Source: CAD feature listing. Evaluate the final solid. Frame: model axes, mm. Give positions to 0.01 mm unless a question says otherwise; leave off trailing zeros. Order: outer loops, then holes, each group sorted by start corner. A loop starts at its lowest first (then second) coordinate and runs counter-clockwise, first axis right, second up.
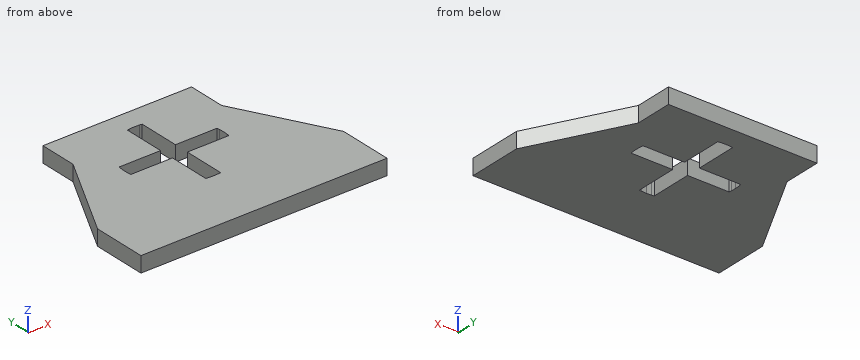
```python
from build123d import *

# Parameters (mm, degrees)
SKETCH1_W           = 49.69
SKETCH1_H           = 27
BOSS_EXTRUDE1_DEPTH = 3.175
CUT_EXTRUDE1_DEPTH  = 3.175
BOSS_EXTRUDE2_DEPTH = 3.175
BOSS_EXTRUDE3_DEPTH = 3.175
CUT_EXTRUDE2_DEPTH  = 3.175
CUT_EXTRUDE3_DEPTH  = 3.175


with BuildPart() as part:
    # Sketch1 → Boss-Extrude1 (new body)
    with BuildSketch(Plane.XY):
        Rectangle(SKETCH1_W, SKETCH1_H)
    extrude(amount=BOSS_EXTRUDE1_DEPTH)

    # Sketch2 → Cut-Extrude1 (cut)
    with BuildSketch(Plane.XY):
        Polygon((10, 6.75), (24.845, -6.75), (24.845, 0), (24.845, 13.5), (10, 13.5), align=None)
        Polygon((-24.845, 13.5), (-24.845, -6.75), (-10, 6.75), (-10, 13.5), align=None)
    extrude(amount=CUT_EXTRUDE1_DEPTH, mode=Mode.SUBTRACT)

    # Sketch3 → Boss-Extrude2 (add)
    with BuildSketch(Plane(origin=(0, 0, 0), x_dir=(-1, 0, 0), z_dir=(0, 0, -1))):
        with BuildLine():
            Line((-24.845, -2.5625), (-24.845, -6.75))
            Line((-24.845, -6.75), (-10, 6.75))
            Line((-10, 6.75), (-10, 13.5))
            Line((-10, 13.5), (-9.028288874, 13.5))
            ThreePointArc((-9.028288874, 13.5), (0, 19.2), (9.028288874, 13.5))
            Line((9.028288874, 13.5), (10, 13.5))
            Line((10, 13.5), (10, 6.75))
            Line((10, 6.75), (24.845, -6.75))
            Line((24.845, -6.75), (24.845, -2.5625))
            Line((24.845, -2.5625), (15, 15.9375))
            Line((15, 15.9375), (15, 23.5))
            Line((15, 23.5), (-15, 23.5))
            Line((-15, 23.5), (-15, 15.9375))
            Line((-15, 15.9375), (-24.845, -2.5625))
        make_face()
    extrude(amount=-BOSS_EXTRUDE2_DEPTH)

    # Sketch4 → Boss-Extrude3 (add)
    # profile 1 of 2: a face of its own
    with BuildSketch(Plane(origin=(0, 0, 0), x_dir=(-1, 0, 0), z_dir=(0, 0, -1))):
        Polygon((-24.845, -2.5625), (-24.845, -13.5), (0, -13.5), (24.845, -13.5), (24.845, -2.5625), (15, 15.9375), (15, 23.5), (-15, 23.5), (-15, 15.9375), align=None)
        with BuildLine():
            ThreePointArc((10, 9.2), (7.071067812, 2.128932188), (0, -0.8))
            ThreePointArc((0, -0.8), (-8.455767263, 3.861460874), (-9.028288874, 13.5))
            ThreePointArc((-9.028288874, 13.5), (0, 19.2), (9.028288874, 13.5))
            ThreePointArc((9.028288874, 13.5), (9.754047589, 11.404213154), (10, 9.2))
        make_face(mode=Mode.SUBTRACT)
    # profile 2 of 2: a face of its own
    with BuildSketch(Plane(origin=(0, 0, 0), x_dir=(-1, 0, 0), z_dir=(0, 0, -1))):
        with BuildLine():
            ThreePointArc((-9.028288874, 13.5), (0, 19.2), (9.028288874, 13.5))
            Line((9.028288874, 13.5), (-9.028288874, 13.5))
        make_face()
    extrude(amount=-BOSS_EXTRUDE3_DEPTH)

    # Sketch5 → Cut-Extrude2 (cut)
    with BuildSketch(Plane(origin=(0, 0, 0), x_dir=(-1, 0, 0), z_dir=(0, 0, -1))):
        with BuildLine():
            Line((9.949874371, 10.2), (1, 10.2))
            Line((1, 10.2), (1, 19.149874371))
            ThreePointArc((1, 19.149874371), (0, 19.2), (-1, 19.149874371))
            Line((-1, 19.149874371), (-1, 10.2))
            Line((-1, 10.2), (-9.949874371, 10.2))
            ThreePointArc((-9.949874371, 10.2), (-10, 9.2), (-9.949874371, 8.2))
            Line((-9.949874371, 8.2), (-1, 8.2))
            Line((-1, 8.2), (-1, -0.749874371))
            ThreePointArc((-1, -0.749874371), (-0.500627751, -0.787460731), (0, -0.8))
            ThreePointArc((0, -0.8), (0.500627751, -0.787460731), (1, -0.749874371))
            Line((1, -0.749874371), (1, 8.2))
            Line((1, 8.2), (9.949874371, 8.2))
            ThreePointArc((9.949874371, 8.2), (9.987460731, 8.699372249), (10, 9.2))
            ThreePointArc((10, 9.2), (9.987460731, 9.700627751), (9.949874371, 10.2))
        make_face()
    extrude(amount=-CUT_EXTRUDE2_DEPTH, mode=Mode.SUBTRACT)

    # Sketch6 → Cut-Extrude3 (cut)
    with BuildSketch(Plane(origin=(0, 0, 0), x_dir=(-1, 0, 0), z_dir=(0, 0, -1))):
        with BuildLine():
            Line((1.5, 10.7), (1.5, 19.086859967))
            ThreePointArc((1.5, 19.086859967), (1.250397018, 19.121517389), (1, 19.149874371))
            Line((1, 19.149874371), (1, 10.2))
            Line((1, 10.2), (9.949874371, 10.2))
            ThreePointArc((9.949874371, 10.2), (9.921517389, 10.450397018), (9.886859967, 10.7))
            Line((9.886859967, 10.7), (1.5, 10.7))
        make_face()
        with BuildLine():
            Line((-1, 10.2), (-1, 19.149874371))
            ThreePointArc((-1, 19.149874371), (-1.250397018, 19.121517389), (-1.5, 19.086859967))
            Line((-1.5, 19.086859967), (-1.5, 10.7))
            Line((-1.5, 10.7), (-9.886859967, 10.7))
            ThreePointArc((-9.886859967, 10.7), (-9.921517389, 10.450397018), (-9.949874371, 10.2))
            Line((-9.949874371, 10.2), (-1, 10.2))
        make_face()
        with BuildLine():
            ThreePointArc((9.886859967, 7.7), (9.921517389, 7.949602982), (9.949874371, 8.2))
            Line((9.949874371, 8.2), (1, 8.2))
            Line((1, 8.2), (1, -0.749874371))
            ThreePointArc((1, -0.749874371), (1.250397018, -0.721517389), (1.5, -0.686859967))
            Line((1.5, -0.686859967), (1.5, 7.7))
            Line((1.5, 7.7), (9.886859967, 7.7))
        make_face()
        with BuildLine():
            Line((-1, -0.749874371), (-1, 8.2))
            Line((-1, 8.2), (-9.949874371, 8.2))
            ThreePointArc((-9.949874371, 8.2), (-9.921517389, 7.949602982), (-9.886859967, 7.7))
            Line((-9.886859967, 7.7), (-1.5, 7.7))
            Line((-1.5, 7.7), (-1.5, -0.686859967))
            ThreePointArc((-1.5, -0.686859967), (-1.250397018, -0.721517389), (-1, -0.749874371))
        make_face()
    extrude(amount=-CUT_EXTRUDE3_DEPTH, mode=Mode.SUBTRACT)


solid = part.part
```
1) Section query C-C, the plane y = 17. Return the cut outline in (x, z) (3 decimals), and give its area (3 significant figures).
Report:
outline: (-15, 0) - (-1.5, 0) - (-1.5, 3.175) - (-15, 3.175) - close; (1.5, 0) - (15, 0) - (15, 3.175) - (1.5, 3.175) - close
area: 85.7 mm2
2) Section query B-B, the plane z = 0.7. Return the cut outline in (x, y) (1 decimal), and give its area (3 significant figures).
Report:
outline: (-24.8, -13.5) - (24.8, -13.5) - (24.8, -2.6) - (15, 15.9) - (15, 23.5) - (-15, 23.5) - (-15, 15.9) - (-24.8, -2.6) - close; hole (-9.9, 7.7) - (-1.5, 7.7) - (-1.5, -0.7) arc R10 ccw to (1.5, -0.7) - (1.5, 7.7) - (9.9, 7.7) arc R10 ccw to (9.9, 10.7) - (1.5, 10.7) - (1.5, 19.1) arc R10 ccw to (-1.5, 19.1) - (-1.5, 10.7) - (-9.9, 10.7) arc R10 ccw to start
area: 1,400 mm2
3) Material intervals for L1, parallel to Y at x = 1, z = 1.85; L2, parallel to Y at x = 4, z = 1.75; L3, parallel to X at y = 19, z = 0.9, sorted ascending.
Report:
L1: y = -13.5 to -0.75, 19.15 to 23.5
L2: y = -13.5 to 7.7, 10.7 to 23.5
L3: x = -15 to -1.5, 1.5 to 15
4) Pin query (flat end, axial travel): pin 1 (1.6 mm diameter, centred on y = 5.5, z = 2, fed in from +X); pin 2 (1 mm diameter, centred on y = 15, z = 1.5, fed in from -X) (3 decimals); pin 3 (1 mm diameter, centred on y = 20.5, z = 1, fed in from -X). Return the tip coordinate at first contact, or that it passes through.
Report:
pin 1: stops at x = 20.98
pin 2: stops at x = -15.765
pin 3: stops at x = -15
5) Section query D-D, the plane x = -21. Return the cut outline in (y, z) (3 decimals).
Report:
outline: (-13.5, 0) - (4.663, 0) - (4.663, 3.175) - (-13.5, 3.175) - close
6) Section query A-A, the plane x = 9. Return the cut outline in (y, z) (3 decimals).
Report:
outline: (-13.5, 0) - (7.7, 0) - (7.7, 3.175) - (-13.5, 3.175) - close; (10.7, 0) - (23.5, 0) - (23.5, 3.175) - (10.7, 3.175) - close
